from build123d import *

# Parameters (mm, degrees)
ESQUISSE2_W                            = 330
ESQUISSE2_H                            = 340
BOSS_EXTRU_1_DEPTH                     = 6
ESQUISSE4_W                            = 65
ESQUISSE4_H                            = 6
ESQUISSE4_W_2                          = 40
ESQUISSE4_W_3                          = 6
ESQUISSE4_H_2                          = 68
ENL_V_MAT_ENCOCHE_BORD_DEPTH           = 474.852297662
ESQUISSE5_W                            = 38
ESQUISSE5_H                            = 6
ESQUISSE5_W_2                          = 15
ESQUISSE5_H_2                          = 10
ESQUISSE5_W_3                          = 25
ESQUISSE5_H_3                          = 30
ESQUISSE5_W_4                          = 20
ESQUISSE5_W_5                          = 6
ESQUISSE5_H_4                          = 20
ENL_V_MAT_ENCOCHE_TAGE_ROULETTES_DEPTH = 474.852297662
ESQUISSE6_R                            = 8
ENL_V_MAT_EXTRU_1_DEPTH                = 10
ESQUISSE7_W                            = 170.318171934
ESQUISSE7_H                            = 348.032193401
ENL_V_MAT_EXTRU_2_DEPTH                = 474.852297662
ESQUISSE8_R                            = 1.5
ENL_V_MAT_EXTRU_3_DEPTH                = 378.969575495
ESQUISSE9_R                            = 2.995
ESQUISSE9_R_2                          = 3
ENL_V_MAT_EXTRU_4_DEPTH                = 3


with BuildPart() as part:
    # Esquisse2 → Boss.-Extru.1 (new body)
    with BuildSketch(Plane.XY):
        with Locations((-165, -170)):
            Rectangle(ESQUISSE2_W, ESQUISSE2_H)
    extrude(amount=BOSS_EXTRU_1_DEPTH)

    # Esquisse4 → Enlèv. mat encoche bord (cut, through all)
    with BuildSketch(Plane(origin=(0, 0, 0), x_dir=(-1, 0, 0), z_dir=(0, 0, -1))):
        with Locations((297.5, -3)):
            Rectangle(ESQUISSE4_W, ESQUISSE4_H)
        with Locations((205, -3)):
            Rectangle(ESQUISSE4_W_2, ESQUISSE4_H)
        with Locations((125, -3)):
            Rectangle(ESQUISSE4_W_2, ESQUISSE4_H)
        with Locations((32.5, -3)):
            Rectangle(ESQUISSE4_W, ESQUISSE4_H)
        with Locations((327, -102)):
            Rectangle(ESQUISSE4_W_3, ESQUISSE4_H_2)
        with Locations((3, -102)):
            Rectangle(ESQUISSE4_W_3, ESQUISSE4_H_2)
        with Locations((297.5, -337)):
            Rectangle(ESQUISSE4_W, ESQUISSE4_H)
        with Locations((205, -337)):
            Rectangle(ESQUISSE4_W_2, ESQUISSE4_H)
        with Locations((125, -337)):
            Rectangle(ESQUISSE4_W_2, ESQUISSE4_H)
        with Locations((32.5, -337)):
            Rectangle(ESQUISSE4_W, ESQUISSE4_H)
        with Locations((327, -238)):
            Rectangle(ESQUISSE4_W_3, ESQUISSE4_H_2)
        with Locations((3, -238)):
            Rectangle(ESQUISSE4_W_3, ESQUISSE4_H_2)
    extrude(amount=-ENL_V_MAT_ENCOCHE_BORD_DEPTH, mode=Mode.SUBTRACT)

    # Esquisse5 → Enlèv. mat encoche étage + roulettes (cut, through all)
    with BuildSketch(Plane(origin=(0, 0, 0), x_dir=(-1, 0, 0), z_dir=(0, 0, -1))):
        with Locations((251, -273)):
            Rectangle(ESQUISSE5_W, ESQUISSE5_H)
        with Locations((79, -273)):
            Rectangle(ESQUISSE5_W, ESQUISSE5_H)
        with Locations((322.5, -11)):
            Rectangle(ESQUISSE5_W_2, ESQUISSE5_H_2)
        with Locations((12.5, -21)):
            Rectangle(ESQUISSE5_W_3, ESQUISSE5_H_3)
        with Locations((300, -99)):
            Rectangle(ESQUISSE5_W_4, ESQUISSE5_H)
        with Locations((30, -99)):
            Rectangle(ESQUISSE5_W_4, ESQUISSE5_H)
        with Locations((53, -305)):
            Rectangle(ESQUISSE5_W_5, ESQUISSE5_H_4)
    extrude(amount=-ENL_V_MAT_ENCOCHE_TAGE_ROULETTES_DEPTH, mode=Mode.SUBTRACT)

    # Esquisse6 → Enlèv. mat.-Extru.1 (cut)
    with BuildSketch(Plane.XY.offset(6)):
        with Locations((-21, -178.92)):
            Circle(ESQUISSE6_R)
        with Locations((-309, -178.92)):
            Circle(ESQUISSE6_R)
    extrude(amount=-ENL_V_MAT_EXTRU_1_DEPTH, mode=Mode.SUBTRACT)

    # Esquisse7 → Enlèv. mat.-Extru.2 (cut, through all)
    with BuildSketch(Plane.XY.offset(6)):
        with Locations((-250.159085967, -174.016096701)):
            Rectangle(ESQUISSE7_W, ESQUISSE7_H)
    extrude(amount=-ENL_V_MAT_EXTRU_2_DEPTH, mode=Mode.SUBTRACT)

    # Esquisse8 → Enlèv. mat.-Extru.3 (cut, through all)
    with BuildSketch(Plane(origin=(0, 0, 0), x_dir=(-1, 0, 0), z_dir=(0, 0, -1))):
        with Locations((155, -337)):
            Circle(ESQUISSE8_R)
        with Locations((98, -337)):
            Circle(ESQUISSE8_R)
        with Locations((72, -337)):
            Circle(ESQUISSE8_R)
        with Locations((3, -327)):
            Circle(ESQUISSE8_R)
        with Locations((3, -303)):
            Circle(ESQUISSE8_R)
        with Locations((3, -279)):
            Circle(ESQUISSE8_R)
        with Locations((53, -288)):
            Circle(ESQUISSE8_R)
        with Locations((53, -322)):
            Circle(ESQUISSE8_R)
        with Locations((53, -273)):
            Circle(ESQUISSE8_R)
        with Locations((105, -273)):
            Circle(ESQUISSE8_R)
        with Locations((3, -197)):
            Circle(ESQUISSE8_R)
        with Locations((3, -170)):
            Circle(ESQUISSE8_R)
        with Locations((3, -143)):
            Circle(ESQUISSE8_R)
        with Locations((3, -61)):
            Circle(ESQUISSE8_R)
        with Locations((3, -43)):
            Circle(ESQUISSE8_R)
        with Locations((98, -3)):
            Circle(ESQUISSE8_R)
        with Locations((72, -3)):
            Circle(ESQUISSE8_R)
        with Locations((155, -3)):
            Circle(ESQUISSE8_R)
        with Locations((47, -99)):
            Circle(ESQUISSE8_R)
        with Locations((13, -99)):
            Circle(ESQUISSE8_R)
    extrude(amount=-ENL_V_MAT_EXTRU_3_DEPTH, mode=Mode.SUBTRACT)

    # Esquisse9 → Enlèv. mat.-Extru.4 (cut)
    with BuildSketch(Plane(origin=(0, 0, 0), x_dir=(-1, 0, 0), z_dir=(0, 0, -1))):
        with Locations((155, -337)):
            Circle(ESQUISSE9_R)
        with Locations((98, -337)):
            Circle(ESQUISSE9_R)
        with Locations((72, -337)):
            Circle(ESQUISSE9_R)
        with Locations((53, -322)):
            Circle(ESQUISSE9_R_2)
        with Locations((53, -288)):
            Circle(ESQUISSE9_R)
        with Locations((53, -273)):
            Circle(ESQUISSE9_R)
        with Locations((105, -273)):
            Circle(ESQUISSE9_R)
        with Locations((3, -279)):
            Circle(ESQUISSE9_R)
        with Locations((3, -303)):
            Circle(ESQUISSE9_R)
        with Locations((3, -327)):
            Circle(ESQUISSE9_R)
        with Locations((3, -197)):
            Circle(ESQUISSE9_R)
        with Locations((3, -170)):
            Circle(ESQUISSE9_R)
        with Locations((3, -143)):
            Circle(ESQUISSE9_R)
        with Locations((47, -99)):
            Circle(ESQUISSE9_R_2)
        with Locations((13, -99)):
            Circle(ESQUISSE9_R_2)
        with Locations((3, -61)):
            Circle(ESQUISSE9_R)
        with Locations((3, -43)):
            Circle(ESQUISSE9_R)
        with Locations((98, -3)):
            Circle(ESQUISSE9_R)
        with Locations((72, -3)):
            Circle(ESQUISSE9_R)
        with Locations((155, -3)):
            Circle(ESQUISSE9_R)
    extrude(amount=-ENL_V_MAT_EXTRU_4_DEPTH, mode=Mode.SUBTRACT)


solid = part.part
Geometry: final body of the model. Coordinates: model frame, mm. A direction names the side the tool comes from. Round coordinates to 2 decimals unless told otherwise and drop trailing zeros. Order: outer loops, then holes, each group sorted by start corner. A loop starts at its lowest first (then second) coordinate and runs counter-clockwise, first axis right, second up. Notation, with made-up numbers: (41.5, 50.25) - (47.5, 50.25) arc R33 ccw to (47.5, 89.25) - close; hole circle Ø6 at (79.25, 12). An arc over 180 degrees is marked (long way). Write each question's results on one line, items separated by ' | '.
Item 1: First-contact query: pin 1 Ø5 at (x, y) = (-13, -99) entering from +Z; pin 2 Ø4 at (x, y) = (-105, -273) entering from -Z; pin 3 Ø1.8 at (x, z) = (-2, 4) entering from +Y. Flat tips, straight axial feed; report the tip coordinate or a pass-through.
Completed:
pin 1: z = 6 | pin 2: z = 3 | pin 3: y = -36
Item 2: Section D-D, the plane x = -79. Return the cut outline in (y, z).
Completed:
outline: (-340, 0) - (-276, 0) - (-276, 6) - (-340, 6) - close; (-270, 0) - (0, 0) - (0, 6) - (-270, 6) - close
Item 3: Material intervals for line 1 along Y through (x, z) = (-69.5, 5.75); line 2 along X through (y, z) = (-260.5, 4.1); line 3 along Y through (x, z) = (-74.5, 1.3), sorted ascending. Write a range as [from, to].
Completed:
line 1: [-340, -276], [-270, 0] | line 2: [-165, -6] | line 3: [-340, -338.65], [-335.35, -276], [-270, -4.65], [-1.35, 0]
Item 4: Mould query, pull axis X, two halves, no side actions, for faces 1 (the flat face through (-45, -6, 3)), 2 (the cylindrical face through (-53, -319, 1)), 3 (the flat face through (-165, -172, 3)). Classes: pulls with the +X half, pulls with the -X half, needs draft (parallel to the pull), parting line crosses it, or undercut.
Completed:
face 1: needs draft | face 2: undercut | face 3: pulls with the -X half
Item 5: Reachability of faces 4 (the flat face through (-3, -136, 3)), 5 (the flat face through (-106.3, -274.3, 3)), 6 (the flat face through (-30, -102, 3)), 7 (the flat face through (-105, -3, 3)), 8 (the flat face through (-65, -337, 3)) from +Z, -Z, +X, -X, +Y, -Y: full face, straight path, thin tool, end or side. Return the list, or none.
Completed:
face 4: +Z, -Z, +X | face 5: -Z | face 6: +Z, -Z | face 7: +Z, -Z, +Y | face 8: +Z, -Z, +X, -Y
Item 6: Section C-C, the plane y = -89.5. Return the cut outline in (x, z).
Completed:
outline: (-165, 0) - (-6, 0) - (-6, 6) - (-165, 6) - close
Item 7: Section B-B, the plane z = 4.6. State how many separate pieces and enclosed holes the cut face has, and give its area (3 significant figures).
Completed:
separate pieces: 1 | enclosed holes: 24 | area: 52,500 mm^2
Item 8: Section A-A, the plane x = -36. Return the cut outline in (y, z).
Completed:
outline: (-334, 0) - (-102, 0) - (-102, 6) - (-334, 6) - close; (-96, 0) - (-6, 0) - (-6, 6) - (-96, 6) - close
